Autodesk Inventor part; units mm, degrees
ref_plane "YZ Plane" through (0, 0, 0) normal (1, 0, 0) x (0, 1, 0)
ref_plane "XZ Plane" through (0, 0, 0) normal (0, 1, 0) x (-1, 0, 0)
ref_plane "XY Plane" through (0, 0, 0) normal (0, 0, 1) x (1, 0, 0)
sketch "Sketch1" plane through (0, 0, 0) normal (1, 0, 0) x (0, 1, 0)
  circle A0 centre (0, 0) radius 8.5
  line L0 (28.3441, -4) -> (35, -4)
  line L1 (35, 4) -> (35, -4)
  line L2 (28.3441, 4) -> (35, 4)
  circle A1 centre (31.6721, 0) radius 1.625
  line L3 (17.2139, 22.8708) -> (21.9203, 27.5772)
  line L4 (21.9203, 27.5772) -> (27.5772, 21.9203)
  circle A2 centre (22.3955, 22.3955) radius 1.625
  line L5 (22.8708, 17.2139) -> (27.5772, 21.9203)
  line L6 (-4, 28.3441) -> (-4, 35)
  line L7 (-4, 35) -> (4, 35)
  circle A3 centre (0, 31.6721) radius 1.625
  line L8 (4, 28.3441) -> (4, 35)
  line L9 (-22.8708, 17.2139) -> (-27.5772, 21.9203)
  line L10 (-27.5772, 21.9203) -> (-21.9203, 27.5772)
  circle A4 centre (-22.3955, 22.3955) radius 1.625
  line L11 (-17.2139, 22.8708) -> (-21.9203, 27.5772)
  line L12 (-28.3441, -4) -> (-35, -4)
  line L13 (-35, -4) -> (-35, 4)
  circle A5 centre (-31.6721, 0) radius 1.625
  line L14 (-28.3441, 4) -> (-35, 4)
  line L15 (-17.2139, -22.8708) -> (-21.9203, -27.5772)
  line L16 (-21.9203, -27.5772) -> (-27.5772, -21.9203)
  circle A6 centre (-22.3955, -22.3955) radius 1.625
  line L17 (-22.8708, -17.2139) -> (-27.5772, -21.9203)
  line L18 (4, -28.3441) -> (4, -35)
  line L19 (4, -35) -> (-4, -35)
  circle A7 centre (0, -31.6721) radius 1.625
  line L20 (-4, -28.3441) -> (-4, -35)
  line L21 (22.8708, -17.2139) -> (27.5772, -21.9203)
  line L22 (27.5772, -21.9203) -> (21.9203, -27.5772)
  circle A8 centre (22.3955, -22.3955) radius 1.625
  line L23 (17.2139, -22.8708) -> (21.9203, -27.5772)
  arc A9 (22.8708, -17.2139) -> (28.3441, -4) centre (0, 0) ccw
  arc A10 (4, -28.3441) -> (17.2139, -22.8708) centre (0, 0) ccw
  arc A11 (-17.2139, -22.8708) -> (-4, -28.3441) centre (0, 0) ccw
  arc A12 (-28.3441, -4) -> (-22.8708, -17.2139) centre (0, 0) ccw
  arc A13 (-22.8708, 17.2139) -> (-28.3441, 4) centre (0, 0) ccw
  arc A14 (-4, 28.3441) -> (-17.2139, 22.8708) centre (0, 0) ccw
  arc A15 (28.3441, 4) -> (22.8708, 17.2139) centre (0, 0) ccw
  arc A16 (17.2139, 22.8708) -> (4, 28.3441) centre (0, 0) ccw
  dimension "d0" = 17
  dimension "d8" = 360
  dimension "d12" = 3.25
extrude "Extrusion1" add sketch "Sketch1" along normal blind 3
sketch "Sketch2" plane through (3, 0, 0) normal (1, 0, 0) x (0, 0, -1)
  line L0 (-5.2542, 23.7941) -> (-5.2542, 26.8421)
  line L1 (-5.2542, 26.8421) -> (-2.9174, 26.8421)
  line L2 (-2.9174, 26.8421) -> (-2.9174, 26.5373)
  line L3 (-2.9174, 26.5373) -> (-4.9494, 26.5373)
  line L4 (-4.9494, 26.5373) -> (-4.9494, 25.5721)
  line L5 (-4.9494, 25.5721) -> (-2.9174, 25.5721)
  line L6 (-2.9174, 25.5721) -> (-2.9174, 25.2673)
  line L7 (-2.9174, 25.2673) -> (-4.9494, 25.2673)
  line L8 (-4.9494, 25.2673) -> (-4.9494, 23.7941)
  line L9 (-4.9494, 23.7941) -> (-5.2542, 23.7941)
  line L10 (-5.2034, 23.8449) -> (-5.2034, 26.7913)
  line L11 (-5.2034, 26.7913) -> (-2.9682, 26.7913)
  line L12 (-2.9682, 26.7913) -> (-2.9682, 26.5881)
  line L13 (-2.9682, 26.5881) -> (-5.0002, 26.5881)
  line L14 (-5.0002, 26.5881) -> (-5.0002, 25.5213)
  line L15 (-5.0002, 25.5213) -> (-2.9682, 25.5213)
  line L16 (-2.9682, 25.5213) -> (-2.9682, 25.3181)
  line L17 (-2.9682, 25.3181) -> (-5.0002, 25.3181)
  line L18 (-5.0002, 25.3181) -> (-5.0002, 23.8449)
  line L19 (-5.0002, 23.8449) -> (-5.2034, 23.8449)
  line L20 (-5.1526, 23.8957) -> (-5.1526, 26.7405)
  line L21 (-5.1526, 26.7405) -> (-3.019, 26.7405)
  line L22 (-3.019, 26.7405) -> (-3.019, 26.6389)
  line L23 (-3.019, 26.6389) -> (-5.051, 26.6389)
  line L24 (-5.051, 26.6389) -> (-5.051, 25.4705)
  line L25 (-5.051, 25.4705) -> (-3.019, 25.4705)
  line L26 (-3.019, 25.4705) -> (-3.019, 25.3689)
  line L27 (-3.019, 25.3689) -> (-5.051, 25.3689)
  line L28 (-5.051, 25.3689) -> (-5.051, 23.8957)
  line L29 (-5.051, 23.8957) -> (-5.1526, 23.8957)
  line L30 (-5.1018, 23.9465) -> (-5.1018, 26.6897)
  line L31 (-5.1018, 26.6897) -> (-3.0698, 26.6897)
  line L32 (-3.0698, 25.4197) -> (-5.1018, 25.4197)
  line L33 (-2.511, 23.7941) -> (-2.511, 26.0293)
  line L34 (-2.511, 26.0293) -> (-2.2062, 26.0293)
  line L35 (-2.2062, 26.0293) -> (-2.2062, 25.6737)
  arc A0 (-1.3889, 26.0291) -> (-2.2062, 25.6737) centre (-1.3889, 24.9115) ccw
  line L36 (-1.3889, 26.0291) -> (-1.0841, 26.0291)
  line L37 (-1.0841, 26.0291) -> (-1.0841, 25.7243)
  line L38 (-1.0841, 25.7243) -> (-1.3889, 25.7243)
  arc A1 (-1.3889, 25.7243) -> (-2.2017, 24.9115) centre (-1.3889, 24.9115) ccw
  line L39 (-2.2017, 24.9115) -> (-2.2017, 23.7939)
  line L40 (-2.2017, 23.7939) -> (-2.5065, 23.7939)
  line L41 (-2.4557, 23.8447) -> (-2.4557, 24.9115)
  arc A2 (-1.3889, 25.9783) -> (-2.4557, 24.9115) centre (-1.3889, 24.9115) ccw
  line L42 (-1.3889, 25.9783) -> (-1.1349, 25.9783)
  line L43 (-1.1349, 25.9783) -> (-1.1349, 25.7751)
  line L44 (-1.1349, 25.7751) -> (-1.3889, 25.7751)
  arc A3 (-1.3889, 25.7751) -> (-2.2525, 24.9115) centre (-1.3889, 24.9115) ccw
  line L45 (-2.2525, 24.9115) -> (-2.2525, 23.8447)
  line L46 (-2.2525, 23.8447) -> (-2.4557, 23.8447)
  line L47 (-2.4049, 23.8955) -> (-2.4049, 24.9115)
  arc A4 (-1.3889, 25.9275) -> (-2.4049, 24.9115) centre (-1.3889, 24.9115) ccw
  line L48 (-1.3889, 25.9275) -> (-1.1857, 25.9275)
  line L49 (-1.1857, 25.9275) -> (-1.1857, 25.8259)
  line L50 (-1.1857, 25.8259) -> (-1.3889, 25.8259)
  arc A5 (-1.3889, 25.8259) -> (-2.3033, 24.9115) centre (-1.3889, 24.9115) ccw
  line L51 (-2.3033, 24.9115) -> (-2.3033, 23.8955)
  line L52 (-2.3033, 23.8955) -> (-2.4049, 23.8955)
  line L53 (-2.3541, 23.9463) -> (-2.3541, 24.9115)
  arc A6 (-1.3889, 25.8767) -> (-2.3541, 24.9115) centre (-1.3889, 24.9115) ccw
  line L54 (-1.3889, 25.8767) -> (-1.2365, 25.8767)
  line L55 (-2.4557, 24.9115) -> (-2.4557, 25.9783)
  line L56 (-2.4557, 25.9783) -> (-2.2525, 25.9783)
  line L57 (-2.2525, 25.9783) -> (-2.2525, 25.5211)
  line L58 (-2.3033, 25.4703) -> (-2.3033, 25.9275)
  line L59 (-2.3033, 25.9275) -> (-2.4049, 25.9275)
  line L60 (-2.4049, 25.9275) -> (-2.4049, 25.2163)
  line L61 (-2.3541, 25.3687) -> (-2.3541, 25.8767)
  circle A7 centre (0.4399, 24.9115) radius 1.1176
  circle A8 centre (0.4399, 24.9115) radius 0.8128
  circle A9 centre (0.4399, 24.9115) radius 0.8636
  circle A10 centre (0.4399, 24.9115) radius 0.9144
  circle A11 centre (0.4399, 24.9115) radius 0.9652
  circle A12 centre (0.4399, 24.9115) radius 1.016
  circle A13 centre (0.4399, 24.9115) radius 1.0668
  line L62 (1.9639, 23.7939) -> (1.9639, 26.0291)
  line L63 (1.9639, 26.0291) -> (2.2687, 26.0291)
  line L64 (2.2687, 26.0291) -> (2.2687, 25.8005)
  arc A14 (3.795, 25.121) -> (2.2687, 25.8005) centre (2.8806, 25.121) ccw
  line L65 (3.795, 25.121) -> (3.795, 23.8002)
  line L66 (3.795, 23.8002) -> (3.4902, 23.8002)
  line L67 (3.4902, 23.8002) -> (3.4902, 25.121)
  arc A15 (3.4902, 25.121) -> (2.271, 25.121) centre (2.8806, 25.121) ccw
  line L68 (2.271, 25.121) -> (2.271, 23.8002)
  line L69 (2.271, 23.8002) -> (1.9662, 23.8002)
  line L70 (2.017, 23.851) -> (2.017, 25.121)
  arc A16 (3.7442, 25.121) -> (2.017, 25.121) centre (2.8806, 25.121) ccw
  line L71 (3.7442, 25.121) -> (3.7442, 23.851)
  line L72 (3.7442, 23.851) -> (3.541, 23.851)
  line L73 (3.541, 23.851) -> (3.541, 25.121)
  arc A17 (3.541, 25.121) -> (2.2202, 25.121) centre (2.8806, 25.121) ccw
  line L74 (2.2202, 25.121) -> (2.2202, 23.851)
  line L75 (2.2202, 23.851) -> (2.017, 23.851)
  line L76 (2.0678, 23.9018) -> (2.0678, 25.121)
  arc A18 (3.6934, 25.121) -> (2.0678, 25.121) centre (2.8806, 25.121) ccw
  line L77 (3.6934, 25.121) -> (3.6934, 23.9018)
  line L78 (3.6934, 23.9018) -> (3.5918, 23.9018)
  line L79 (3.5918, 23.9018) -> (3.5918, 25.121)
  arc A19 (3.5918, 25.121) -> (2.1694, 25.121) centre (2.8806, 25.121) ccw
  line L80 (2.1694, 25.121) -> (2.1694, 23.9018)
  line L81 (2.1694, 23.9018) -> (2.0678, 23.9018)
  line L82 (2.1186, 23.9526) -> (2.1186, 25.121)
  arc A20 (3.6426, 25.121) -> (2.1186, 25.121) centre (2.8806, 25.121) ccw
  line L83 (3.6426, 25.121) -> (3.6426, 23.9526)
  line L84 (2.017, 25.121) -> (2.017, 25.9846)
  line L85 (2.017, 25.9846) -> (2.2202, 25.9846)
  line L86 (2.2202, 25.9846) -> (2.2202, 25.6798)
  line L87 (2.1694, 25.629) -> (2.1694, 25.9338)
  line L88 (2.1694, 25.9338) -> (2.0678, 25.9338)
  line L89 (2.0678, 25.9338) -> (2.0678, 25.375)
  line L90 (2.1186, 25.5274) -> (2.1186, 25.883)
  arc A21 (4.4554, 24.2066) -> (4.8618, 23.8002) centre (4.8618, 24.2066) ccw
  line L91 (4.4554, 24.2066) -> (4.4554, 25.7306)
  line L92 (4.4554, 25.7306) -> (4.1506, 25.7306)
  line L93 (4.1506, 25.7306) -> (4.1506, 26.0354)
  line L94 (4.1506, 26.0354) -> (4.4554, 26.0354)
  line L95 (4.4554, 26.0354) -> (4.4554, 26.8482)
  line L96 (4.4554, 26.8482) -> (4.7602, 26.8482)
  line L97 (4.7602, 26.8482) -> (4.7602, 26.0354)
  line L98 (4.7602, 26.0354) -> (5.065, 26.0354)
  line L99 (5.065, 26.0354) -> (5.065, 25.7306)
  line L100 (5.065, 25.7306) -> (4.7602, 25.7306)
  line L101 (4.7602, 25.7306) -> (4.7602, 24.2066)
  arc A22 (4.7602, 24.2066) -> (4.8618, 24.105) centre (4.8618, 24.2066) ccw
  line L102 (4.8618, 24.105) -> (5.065, 24.105)
  line L103 (5.065, 24.105) -> (5.065, 23.8002)
  line L104 (5.065, 23.8002) -> (4.8618, 23.8002)
  arc A23 (4.5062, 24.2066) -> (4.8618, 23.851) centre (4.8618, 24.2066) ccw
  line L105 (4.5062, 24.2066) -> (4.5062, 25.7814)
  line L106 (4.5062, 25.7814) -> (4.2014, 25.7814)
  line L107 (4.2014, 25.7814) -> (4.2014, 25.9846)
  line L108 (4.2014, 25.9846) -> (4.5062, 25.9846)
  line L109 (4.5062, 25.9846) -> (4.5062, 26.7974)
  line L110 (4.5062, 26.7974) -> (4.7094, 26.7974)
  line L111 (4.7094, 26.7974) -> (4.7094, 25.9846)
  line L112 (4.7094, 25.9846) -> (5.0142, 25.9846)
  line L113 (5.0142, 25.9846) -> (5.0142, 25.7814)
  line L114 (5.0142, 25.7814) -> (4.7094, 25.7814)
  line L115 (4.7094, 25.7814) -> (4.7094, 24.2066)
  arc A24 (4.7094, 24.2066) -> (4.8618, 24.0542) centre (4.8618, 24.2066) ccw
  line L116 (4.8618, 24.0542) -> (5.0142, 24.0542)
  line L117 (5.0142, 24.0542) -> (5.0142, 23.851)
  line L118 (5.0142, 23.851) -> (4.8618, 23.851)
  arc A25 (4.557, 24.2066) -> (4.8618, 23.9018) centre (4.8618, 24.2066) ccw
  line L119 (4.557, 24.2066) -> (4.557, 25.8322)
  line L120 (4.557, 25.8322) -> (4.2522, 25.8322)
  line L121 (4.2522, 25.8322) -> (4.2522, 25.9338)
  line L122 (4.2522, 25.9338) -> (4.557, 25.9338)
  line L123 (4.557, 25.9338) -> (4.557, 26.7466)
  line L124 (4.557, 26.7466) -> (4.6586, 26.7466)
  line L125 (4.6586, 26.7466) -> (4.6586, 25.9338)
  line L126 (4.6586, 25.9338) -> (4.9634, 25.9338)
  line L127 (4.9634, 25.9338) -> (4.9634, 25.8322)
  line L128 (4.9634, 25.8322) -> (4.6586, 25.8322)
  line L129 (4.6586, 25.8322) -> (4.6586, 24.2066)
  arc A26 (4.6586, 24.2066) -> (4.8618, 24.0034) centre (4.8618, 24.2066) ccw
  line L130 (4.8618, 24.0034) -> (4.9634, 24.0034)
  line L131 (4.9634, 24.0034) -> (4.9634, 23.9018)
  line L132 (4.9634, 23.9018) -> (4.8618, 23.9018)
  line L133 (4.9126, 23.9526) -> (4.8618, 23.9526)
  arc A27 (4.6078, 24.2066) -> (4.8618, 23.9526) centre (4.8618, 24.2066) ccw
  line L134 (4.6078, 24.2066) -> (4.6078, 26.6958)
  line L135 (4.303, 25.883) -> (4.9126, 25.883)
  point P0 (0, 0)
  point P1 (-2.2525, 25.5378)
extrude "Extrusion2" [suppressed]
chamfer "Chamfer1" distance 1.1 angle 45 8 edges at (3, 30.0471, 0) (3, 20.7705, -22.3955) (3, -1.625, -31.6721) (3, -24.0205, -22.3955) (3, -33.2971, 0) (3, -24.0205, 22.3955) (3, -1.625, 31.6721) (3, 20.7705, 22.3955)
properties part number "Gear_Box_Chasis_Divider" material "ABS Plastic"
The model under review builds one solid part; all positions refer to its coordinate system, in mm. A direction names the side the tool comes from. Give positions to 0.01 mm unless a question says otherwise; leave off trailing zeros. Write each loop counter-clockwise with the first axis right and the second up, starting at its lowest first coordinate (ties: lowest second). Pieces come first, ordered by that corner, then holes. Notation, with made-up numbers: M -32,-35 L -16,-35 A18 cw -16,-9 Z; hole C 78.5,27 d2. An arc over 180 degrees is marked long. One line per question, with ' | ' between items. Start each with the question number.
Item 1: We need section D-D on y = -10. Write out the cut boundary in (x, z), plus the area to 3 significant figures.
Item 2: For pin 1 (1.5 mm diameter, centred on x = 1, y = 30.5, fed in from +Z); pin 2 (5 mm diameter, centred on y = 0, z = 31.67, fed in from +X); pin 3 (1.9 mm diameter, centred on y = 0, z = -31.67, fed in from -X); pin 4 (4 mm diameter, centred on y = -22.4, z = 22.4, fed in from +X), all flat-tipped, find the tip position at first contact; note any pin that passes through.
Item 3: For faces 1 (the flat face through (1, 32, 4)), 2 (the flat face through (1, -4, -32)), 3 (the flat face through (1.479, -25.191, 19.534)), 4 (the flat face through (1.479, -19.534, -25.191)), 5 (the cylindrical face through (1.479, -11.048, 26.407)), list the 3-axis set-ups (+Z, -Z, +X, -X, +Y, -Y) from which the entire face can be reached by the end or side of a thin tool; tool diameter is ignored.
Item 4: Wall thickness on line 1 (Y direction, x = 0.2, z = -31.5); line 2 (Z direction, x = 1.2, y = -22.5); line 3 (Z direction, x = 2.85, y = -24): over which ranges is each line inside the solid? List them lowest first. Write a range as from..to.
Item 5: We need section C-C on x = 0.75. Give the number of separate pieces and of enclosed holes in the cut face, plus the area to 3 significant figures.
Item 6: We need section A-A on y = 0. Write out the cut boundary in (x, z).
Item 7: Draft analysis for pull direction Z (two halves, no side actions). For faces 6 (the flat face through (1, 0, -35)), 7 (the flat face through (1.479, 25.191, -19.534)), 8 (the flat face through (3, 7, -7)), state which applies: released by +Z, released by -Z, zero draft, split by the parting line, or undercut.
Results found:
1) outline: M 0,-26.82 L 3,-26.82 L 3,26.82 L 0,26.82 Z | area: 161 mm2
2) pin 1: stops at z = 4 | pin 2: stops at x = 2.78 | pin 3: passes through | pin 4: stops at x = 2.28
3) face 1: +Z, +X, -X, +Y | face 2: -Z, +X, -X, -Y | face 3: +X, -X, -Y | face 4: -Z, +X, -X | face 5: +Z, +X, -X
4) line 1: y = -4..-1.62, 1.62..4 | line 2: z = -27..-24.02, -20.77..20.77, 24.02..27 | line 3: z = -25.5..-24.41, -20.38..-18.34, -15.6..15.6, 18.34..20.38, 24.41..25.5
5) separate pieces: 1 | enclosed holes: 9 | area: 2,690 mm2
6) outline: M 0,-35 L 3,-35 L 3,-34.4 L 1.9,-33.3 L 0,-33.3 Z; M 0,-30.05 L 1.9,-30.05 L 3,-28.95 L 3,-8.5 L 0,-8.5 Z; M 0,8.5 L 3,8.5 L 3,28.95 L 1.9,30.05 L 0,30.05 Z; M 0,33.3 L 1.9,33.3 L 3,34.4 L 3,35 L 0,35 Z
7) face 6: released by -Z | face 7: undercut | face 8: zero draft
